from build123d import *

# Parameters (mm, degrees)
SKETCH1_R           = 30
SKETCH1_R_2         = 2.5
BOSS_EXTRUDE2_DEPTH = 5
SKETCH2_R           = 10
BOSS_EXTRUDE3_DEPTH = 20
SKETCH3_R           = 5
CUT_EXTRUDE1_DEPTH  = 45


with BuildPart() as part:
    # Sketch1 → Boss-Extrude2 (new body)
    with BuildSketch(Plane(origin=(0, 0, 0), x_dir=(1, 0, 0), z_dir=(0, 1, 0))):
        Circle(SKETCH1_R)
        with Locations((0, 23)):
            Circle(SKETCH1_R_2, mode=Mode.SUBTRACT)
        with Locations((19.918584287, 11.5)):
            Circle(SKETCH1_R_2, mode=Mode.SUBTRACT)
        with Locations((19.918584287, -11.5)):
            Circle(SKETCH1_R_2, mode=Mode.SUBTRACT)
        with Locations((0, -23.561037846)):
            Circle(SKETCH1_R_2, mode=Mode.SUBTRACT)
        with Locations((-19.918584287, -11.5)):
            Circle(SKETCH1_R_2, mode=Mode.SUBTRACT)
        with Locations((-19.918584287, 11.5)):
            Circle(SKETCH1_R_2, mode=Mode.SUBTRACT)
    extrude(amount=BOSS_EXTRUDE2_DEPTH)

    # Sketch2 → Boss-Extrude3 (add)
    with BuildSketch(Plane(origin=(0, 5, 0), x_dir=(1, 0, 0), z_dir=(0, 1, 0))):
        Circle(SKETCH2_R)
    extrude(amount=BOSS_EXTRUDE3_DEPTH)

    # Sketch3 → Cut-Extrude1 (cut)
    with BuildSketch(Plane(origin=(0, 25, 0), x_dir=(1, 0, 0), z_dir=(0, 1, 0))):
        Circle(SKETCH3_R)
    extrude(amount=-CUT_EXTRUDE1_DEPTH, mode=Mode.SUBTRACT)


solid = part.part
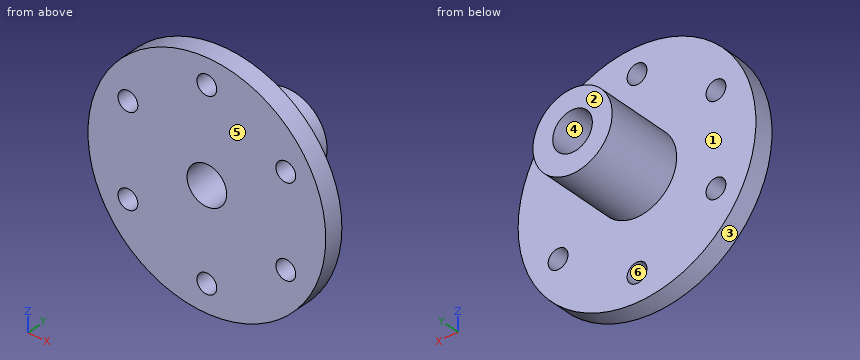
Check sheet for the modelled part. Datum: model origin and axes. Units: mm. Face numbers are marked on the shaded views. A direction names the side the tool comes from. Give positions to 0.01 mm unless a question says otherwise; leave off trailing zeros. Loops run counter-clockwise (first coordinate to the right, second up) from the corner with the lowest first, then second, coordinate; pieces in that order, holes last. Notation, with made-up numbers: M -1,-34.75 L 9,-34.75 A21 cw 9,-27.75 Z; hole C 25,20 d6. An arc over 180 degrees is marked long. Use a Markdown table: item, result. Add a question column.
Q1. Sectioned sample at A-A, the plane z = 0. Record the cut outline in (x, y).
Q2. Sectioned sample at B-B, the plane x = 0. Record the cut outline in (y, z).
Q3. Scan lines: line 1 along Z through (x, y) = (0, 5.5); line 2 along Z through (x, y) = (0, 1.9); line 3 along X through (y, z) = (2.65, -11.5). Record each from-to range of solid material in increasing order. Write a range as [from, to].
Q4. Sectioned sample at C-C, the plane x = -21.5. Record the cut outline in (y, z), then the cut area to 3 significant figures.
Q5. Sectioned sample at D-D, the plane z = 11.5. Record the cut outline in (x, y).
Q6. Tool access check on the marked faces 1 and 2. Record the directions out of +Z, -Z, +X, -X, +Y, -Y that give a thin tool (end or side, any length) a straight path to the whole face; none if there is none.
Q7. Go/stop test with flat-tipped pins: pin 1 (6 mm diameter, centred on x = 0, z = 23.56, fed in from +Y); pin 2 (4 mm diameter, centred on x = 23, y = 6, fed in from -Z); pin 3 (5 mm diameter, centred on y = 21, z = 9.5, fed in from +X). Record where each tip stops, or that it passes through.
Q8. Mould release check, pull along X, two halves, no side actions. Record for the marked faces 3, 4, 5 and 6: pulls with the +X half, pulls with the -X half, needs draft (parallel to the pull), parting line crosses it, or undercut.
Verdict:
| question | item | result |
|---|---|---|
| 1 | outline | M -30,0 L -5,0 L -5,25 L -10,25 L -10,5 L -30,5 Z; M 5,0 L 30,0 L 30,5 L 10,5 L 10,25 L 5,25 Z |
| 2 | outline | M 0,-30 L 5,-30 L 5,-25.5 L 0,-25.5 Z; M 0,-20.5 L 5,-20.5 L 5,-10 L 25,-10 L 25,-5 L 0,-5 Z; M 0,5 L 25,5 L 25,10 L 5,10 L 5,21.06 L 0,21.06 Z; M 0,26.06 L 5,26.06 L 5,30 L 0,30 Z |
| 3 | line 1 | [-10, -5], [5, 10] |
| 3 | line 2 | [-30, -25.5], [-20.5, -5], [5, 21.06], [26.06, 30] |
| 3 | line 3 | [-27.71, -22.42], [-17.42, 17.42], [22.42, 27.71] |
| 4 | outline | M 0,-20.92 L 5,-20.92 L 5,-13.44 L 0,-13.44 Z; M 0,-9.56 L 5,-9.56 L 5,9.56 L 0,9.56 Z; M 0,13.44 L 5,13.44 L 5,20.92 L 0,20.92 Z |
| 4 | area | 170 mm^2 |
| 5 | outline | M -27.71,0 L -22.42,0 L -22.42,5 L -27.71,5 Z; M -17.42,0 L 17.42,0 L 17.42,5 L -17.42,5 Z; M 22.42,0 L 27.71,0 L 27.71,5 L 22.42,5 Z |
| 6 | face 1 | +Y |
| 6 | face 2 | +Z, -Z, +X, -X, +Y |
| 7 | pin 1 | y = 5 |
| 7 | pin 2 | z = -21.16 |
| 7 | pin 3 | x = 7.14 |
| 8 | face 3 | parting line crosses it |
| 8 | face 4 | undercut |
| 8 | face 5 | needs draft |
| 8 | face 6 | undercut |
